The listing builds one solid part. Answer for the finished solid, in the listing's coordinates (mm). Face numbers are marked on the shaded views. A direction names the side the tool comes from. Round coordinates to 2 decimals unless told otherwise and drop trailing zeros. Order: outer loops, then holes, each group sorted by start corner. A loop starts at its lowest first (then second) coordinate and runs counter-clockwise, first axis right, second up. Notation, with made-up numbers: (40.25, 88) -> (57.25, 88) arc R24 ccw to (57.25, 116) -> close; hole circle Ø11 at (46.25, 30.25). An arc over 180 degrees is marked (long way). Answer in a Markdown table with one row per item. Add a question column.
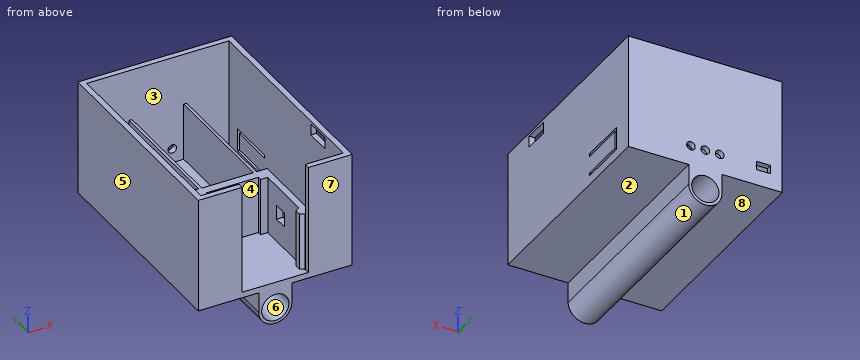
```python
from build123d import *

# Parameters (mm, degrees)
SKETCH1_W            = 25.5
SKETCH1_H            = 72
BOSS_EXTRUDE1_DEPTH  = 2
SKETCH2_W            = 3.75
SKETCH2_H            = 5
SKETCH2_H_2          = 4
BOSS_EXTRUDE2_DEPTH  = 20
SKETCH3_W            = 18
SKETCH3_H            = 3
BOSS_EXTRUDE3_DEPTH  = 20
SKETCH4_W            = 3.75
SKETCH4_H            = 39.4
BOSS_EXTRUDE4_DEPTH  = 20
SKETCH9_W            = 1.25
SKETCH9_H            = 23.6
BOSS_EXTRUDE6_DEPTH  = 20
BOSS_EXTRUDE7_DEPTH  = 20
SKETCH15_W           = 12
SKETCH15_H           = 72
BOSS_EXTRUDE8_DEPTH  = 22
SKETCH16_W           = 53.5
SKETCH16_H           = 76
SKETCH16_W_2         = 49.5
SKETCH16_H_2         = 72
BOSS_EXTRUDE9_DEPTH  = 40
SKETCH17_W           = 9
SKETCH17_H           = 68
CUT_EXTRUDE1_DEPTH   = 20
SKETCH276_R          = 1.5
CUT_EXTRUDE2_DEPTH   = 3
CUT_EXTRUDE3_DEPTH   = 20
CUT_EXTRUDE4_REACH   = 55.5
SKETCH283_W          = 4
SKETCH283_H          = 9
CUT_EXTRUDE5_REACH   = 17.25
SKETCH287_W          = 5
SKETCH287_H          = 5
CUT_EXTRUDE6_REACH   = 42.5
SKETCH288_W          = 5
SKETCH288_H          = 5
CUT_EXTRUDE8_REACH   = 78
SKETCH291_W          = 5
SKETCH291_H          = 3
CUT_EXTRUDE9_REACH   = 55.5
CUT_EXTRUDE10_DEPTH  = 38
SKETCH297_R          = 4.75
BOSS_EXTRUDE10_DEPTH = 76


with BuildPart() as part:
    # Sketch1 → Boss-Extrude1 (new body)
    with BuildSketch(Plane.XY):
        with Locations((-20.131274131, -9.514285714)):
            Rectangle(SKETCH1_W, SKETCH1_H)
    extrude(amount=BOSS_EXTRUDE1_DEPTH)

    # Sketch2 → Boss-Extrude2 (add)
    with BuildSketch(Plane.XY.offset(2)):
        with Locations((-31.006274131, 23.985714286)):
            Rectangle(SKETCH2_W, SKETCH2_H)
        with Locations((-31.006274131, -19.914285714)):
            Rectangle(SKETCH2_W, SKETCH2_H_2)
        with Locations((-9.256274131, -19.914285714)):
            Rectangle(SKETCH2_W, SKETCH2_H_2)
        with Locations((-9.256274131, 23.985714286)):
            Rectangle(SKETCH2_W, SKETCH2_H)
    extrude(amount=BOSS_EXTRUDE2_DEPTH)

    # Sketch3 → Boss-Extrude3 (add)
    with BuildSketch(Plane.XY.offset(2)):
        with Locations((-20.131274131, -19.014285714)):
            Rectangle(SKETCH3_W, SKETCH3_H)
    extrude(amount=BOSS_EXTRUDE3_DEPTH)

    # Sketch4 → Boss-Extrude4 (add)
    with BuildSketch(Plane.XY.offset(2)):
        with Locations((-31.006274131, 1.785714286)):
            Rectangle(SKETCH4_W, SKETCH4_H)
        with Locations((-9.256274131, 1.785714286)):
            Rectangle(SKETCH4_W, SKETCH4_H)
    extrude(amount=BOSS_EXTRUDE4_DEPTH)

    # Sketch9 → Boss-Extrude6 (add)
    with BuildSketch(Plane.XY.offset(2)):
        with Locations((-32.256274131, -33.714285714)):
            Rectangle(SKETCH9_W, SKETCH9_H)
        with Locations((-8.006274131, -33.714285714)):
            Rectangle(SKETCH9_W, SKETCH9_H)
    extrude(amount=BOSS_EXTRUDE6_DEPTH)

    # Sketch11 → Boss-Extrude7 (add)
    with BuildSketch(Plane.XY.offset(2)):
        Polygon((-31.631274131, -45.514285714), (-30.131274131, -44.514285714), (-30.131274131, -42.514285714), (-31.631274131, -41.514285714), align=None)
        Polygon((-8.631274131, -45.514285714), (-10.131274131, -44.514285714), (-10.131274131, -42.514285714), (-8.631274131, -41.514285714), align=None)
    extrude(amount=BOSS_EXTRUDE7_DEPTH)

    # Sketch15 → Boss-Extrude8 (add)
    with BuildSketch(Plane(origin=(0, 0, 0), x_dir=(-1, 0, 0), z_dir=(0, 0, -1))):
        with Locations((38.881274131, -9.514285714)):
            Rectangle(SKETCH15_W, SKETCH15_H)
        with Locations((1.381274131, -9.514285714)):
            Rectangle(SKETCH15_W, SKETCH15_H)
    extrude(amount=-BOSS_EXTRUDE8_DEPTH)

    # Sketch16 → Boss-Extrude9 (add)
    with BuildSketch(Plane(origin=(0, 0, 0), x_dir=(-1, 0, 0), z_dir=(0, 0, -1))):
        with Locations((20.131274131, -9.514285714)):
            Rectangle(SKETCH16_W, SKETCH16_H)
        with Locations((20.131274131, -9.514285714)):
            Rectangle(SKETCH16_W_2, SKETCH16_H_2, mode=Mode.SUBTRACT)
    extrude(amount=-BOSS_EXTRUDE9_DEPTH)

    # Sketch17 → Cut-Extrude1 (cut)
    with BuildSketch(Plane.XY.offset(22)):
        with Locations((-38.381274131, -9.514285714)):
            Rectangle(SKETCH17_W, SKETCH17_H)
        with Locations((-1.881274131, -9.514285714)):
            Rectangle(SKETCH17_W, SKETCH17_H)
    extrude(amount=-CUT_EXTRUDE1_DEPTH, mode=Mode.SUBTRACT)

    # Sketch276 → Cut-Extrude2 (cut, through all)
    with BuildSketch(Plane.XZ.offset(-26.485714286)):
        with Locations((-25.131274131, 7)):
            Circle(SKETCH276_R)
        with Locations((-15.131274131, 7)):
            Circle(SKETCH276_R)
        with Locations((-20.131274131, 7)):
            Circle(SKETCH276_R)
    extrude(amount=-CUT_EXTRUDE2_DEPTH, mode=Mode.SUBTRACT)

    # Sketch282 → Cut-Extrude3 (cut)
    with BuildSketch(Plane.XY.offset(22)):
        Polygon((-33.881274131, -17.418411546), (-30.131274131, -17.418411546), (-30.131274131, 26.485714286), (-44.881274131, 26.485714286), (-44.881274131, -45.514285714), (-33.881274131, -45.514285714), align=None)
        Polygon((-10.131274131, 26.485714286), (-10.131274131, -17.514285714), (-6.381274131, -17.514285714), (-6.381274131, -45.514285714), (4.618725869, -45.514285714), (4.618725869, 26.485714286), align=None)
    extrude(amount=-CUT_EXTRUDE3_DEPTH, mode=Mode.SUBTRACT)

    # Sketch283 → Cut-Extrude4 (cut, up to next)
    with BuildSketch(Plane(origin=(6.618725869, 0, 0), x_dir=(0, 0, -1), z_dir=(1, 0, 0)), mode=Mode.PRIVATE) as cut_extrude4_sk1:
        with Locations((-37, -29.514285714)):
            Rectangle(SKETCH283_W, SKETCH283_H)
    cut_extrude4_tool1 = extrude(cut_extrude4_sk1.sketch, amount=-CUT_EXTRUDE4_REACH, mode=Mode.PRIVATE) & part.part
    add(cut_extrude4_tool1.solids().sort_by_distance((6.618726, -29.514286, 37))[0], mode=Mode.SUBTRACT)

    # Sketch287 → Cut-Extrude5 (cut, up to next)
    with BuildSketch(Plane(origin=(-31.631274131, 0, 0), x_dir=(0, 0, -1), z_dir=(1, 0, 0)), mode=Mode.PRIVATE) as cut_extrude5_sk1:
        with Locations((-12.5, -30.014285714)):
            Rectangle(SKETCH287_W, SKETCH287_H)
    cut_extrude5_tool1 = extrude(cut_extrude5_sk1.sketch, amount=-CUT_EXTRUDE5_REACH, mode=Mode.PRIVATE) & part.part
    add(cut_extrude5_tool1.solids().sort_by_distance((-31.631274, -30.014286, 12.5))[0], mode=Mode.SUBTRACT)

    # Sketch288 → Cut-Extrude6 (cut, up to next)
    with BuildSketch(Plane(origin=(-6.381274131, 0, 0), x_dir=(0, 0, -1), z_dir=(1, 0, 0)), mode=Mode.PRIVATE) as cut_extrude6_sk1:
        with Locations((-12.5, -30.014285714)):
            Rectangle(SKETCH288_W, SKETCH288_H)
    cut_extrude6_tool1 = extrude(cut_extrude6_sk1.sketch, amount=-CUT_EXTRUDE6_REACH, mode=Mode.PRIVATE) & part.part
    add(cut_extrude6_tool1.solids().sort_by_distance((-6.381274, -30.014286, 12.5))[0], mode=Mode.SUBTRACT)

    # Sketch291 → Cut-Extrude8 (cut, up to next)
    with BuildSketch(Plane(origin=(0, 28.485714286, 0), x_dir=(1, 0, 0), z_dir=(0, 1, 0)), mode=Mode.PRIVATE) as cut_extrude8_sk1:
        with Locations((-40.381274131, -7)):
            Rectangle(SKETCH291_W, SKETCH291_H)
    cut_extrude8_tool1 = extrude(cut_extrude8_sk1.sketch, amount=-CUT_EXTRUDE8_REACH, mode=Mode.PRIVATE) & part.part
    add(cut_extrude8_tool1.solids().sort_by_distance((-40.381274, 28.485714, 7))[0], mode=Mode.SUBTRACT)

    # Sketch292 → Cut-Extrude9 (cut, up to next)
    with BuildSketch(Plane(origin=(6.618725869, 0, 0), x_dir=(0, 0, -1), z_dir=(1, 0, 0)), mode=Mode.PRIVATE) as cut_extrude9_sk1:
        Polygon((-10.165543533, 4.001752047), (-11.165543533, 4.001752047), (-11.165543533, 21.001752047), (-3.165543533, 21.001752047), (-3.165543533, 4.001752047), (-4.165543533, 4.001752047), (-4.165543533, 5.001752047), (-4.165543533, 20.001752047), (-10.165543533, 20.001752047), (-10.165543533, 5.001752047), align=None)
    cut_extrude9_tool1 = extrude(cut_extrude9_sk1.sketch, amount=-CUT_EXTRUDE9_REACH, mode=Mode.PRIVATE) & part.part
    add(cut_extrude9_tool1.solids().sort_by_distance((6.618726, 4.189635, 10.665544))[0], mode=Mode.SUBTRACT)

    # Sketch295 → Cut-Extrude10 (cut)
    with BuildSketch(Plane.XY.offset(40)):
        Polygon((-31.631274131, -47.514285714), (-8.614465399, -47.514285714), (-8.614465399, -45.514285714), (-8.631274131, -45.514285714), (-31.631274131, -45.514285714), align=None)
    extrude(amount=-CUT_EXTRUDE10_DEPTH, mode=Mode.SUBTRACT)

    # Sketch297 → Boss-Extrude10 (add)
    with BuildSketch(Plane(origin=(0, 28.485714286, 0), x_dir=(1, 0, 0), z_dir=(0, 1, 0))):
        with BuildLine():
            Line((-25.881274131, 0), (-14.381274131, 0))
            Line((-14.381274131, 0), (-14.381274131, 7.071463376))
            ThreePointArc((-14.381274131, 7.071463376), (-20.131274131, 12.821463376), (-25.881274131, 7.071463376))
            Line((-25.881274131, 7.071463376), (-25.881274131, 0))
        make_face()
        with Locations((-20.131274131, 7.071463376)):
            Circle(SKETCH297_R, mode=Mode.SUBTRACT)
    extrude(amount=-BOSS_EXTRUDE10_DEPTH)


solid = part.part
```
Item 1: A tool of negligible diameter and unlimited length cuts with its end or side. For the marked faces 1, 2, 3, 4 and 5, from which of +Z, -Z, +X, -X, +Y, -Y can it reach the whole face along a straight path? Write none if from no direction.
Item 2: The part is cut by section C-C, the plane z = -5. Give the vertices of the cut face in (x, y).
Item 3: For a pull along Z with two mould halves and no side action, classify the marked faces 6, 7 and 8 as released by +Z, released by -Z, zero draft, split by the parting line, or undercut.
Item 4: The part is cut by section A-A, the plane y = 7.5. State how many separate pieces and enclosed holes the cut face has, and give its area (3 significant figures).
Item 5: The part is cut by section D-D, the plane x = -2.5. Give the vertices of the cut face in (y, z).
Item 6: Find the intervals of material crossed by probe 1 along X at (y, z) = (-20, 11.5); probe 2 along X at (y, z) = (16, 11); probe 3 along Y at (x, z) = (-40, 2.5), in increasing order. Write a range as [from, to].
Item 7: The part is cut by section B-B, the plane x = -42. Give the vertices of the cut face in (y, z).
Item 8: Flat-ended cylindrical pins translate along their axes: P1, Ø4.5, axis at x = -35, y = 3.5, coming from the +Z side; P2, Ø0.6, axis at x = 5.5, y = 12.5, coming from the -Z side; P3, Ø12, axis at x = -21, z = 31.5, coming from the -Y side; P4, Ø8.5, axis at x = -20.13, z = -7.07, coming from the +Y side. Find the tip coordinate at first contact, or state that the pin passes through.
Resolved:
| question | item | result |
|---|---|---|
| 1 | face 1 | -Z, +Y, -Y |
| 1 | face 2 | -Z, +X, +Y, -Y |
| 1 | face 3 | +Z |
| 1 | face 4 | +Z, -Y |
| 1 | face 5 | +Z, -Z, -X, +Y, -Y |
| 2 | outline | (-25.88, -47.51) -> (-24.41, -47.51) -> (-24.41, 28.49) -> (-25.88, 28.49) -> close; (-15.86, -47.51) -> (-14.38, -47.51) -> (-14.38, 28.49) -> (-15.86, 28.49) -> close |
| 3 | face 6 | undercut |
| 3 | face 7 | zero draft |
| 3 | face 8 | released by -Z |
| 4 | separate pieces | 3 |
| 4 | enclosed holes | 1 |
| 4 | area | 357 mm2 |
| 5 | outline | (-47.51, 0) -> (28.49, 0) -> (28.49, 40) -> (26.49, 40) -> (26.49, 2) -> (-45.51, 2) -> (-45.51, 40) -> (-47.51, 40) -> close |
| 6 | probe 1 | [-46.88, -44.88], [-33.88, -6.38], [4.62, 6.62] |
| 6 | probe 2 | [-46.88, -44.88], [-30.13, -29.13], [-11.13, -10.13] |
| 6 | probe 3 | [-47.51, -45.51], [26.49, 28.49] |
| 7 | outline | (-47.51, 0) -> (28.49, 0) -> (28.49, 5.5) -> (26.49, 5.5) -> (26.49, 2) -> (-45.51, 2) -> (-45.51, 40) -> (-47.51, 40) -> close; (26.49, 8.5) -> (28.49, 8.5) -> (28.49, 40) -> (26.49, 40) -> close |
| 8 | P1 | z = 2 |
| 8 | P2 | z = 0 |
| 8 | P3 | y = 26.49 |
| 8 | P4 | through |
